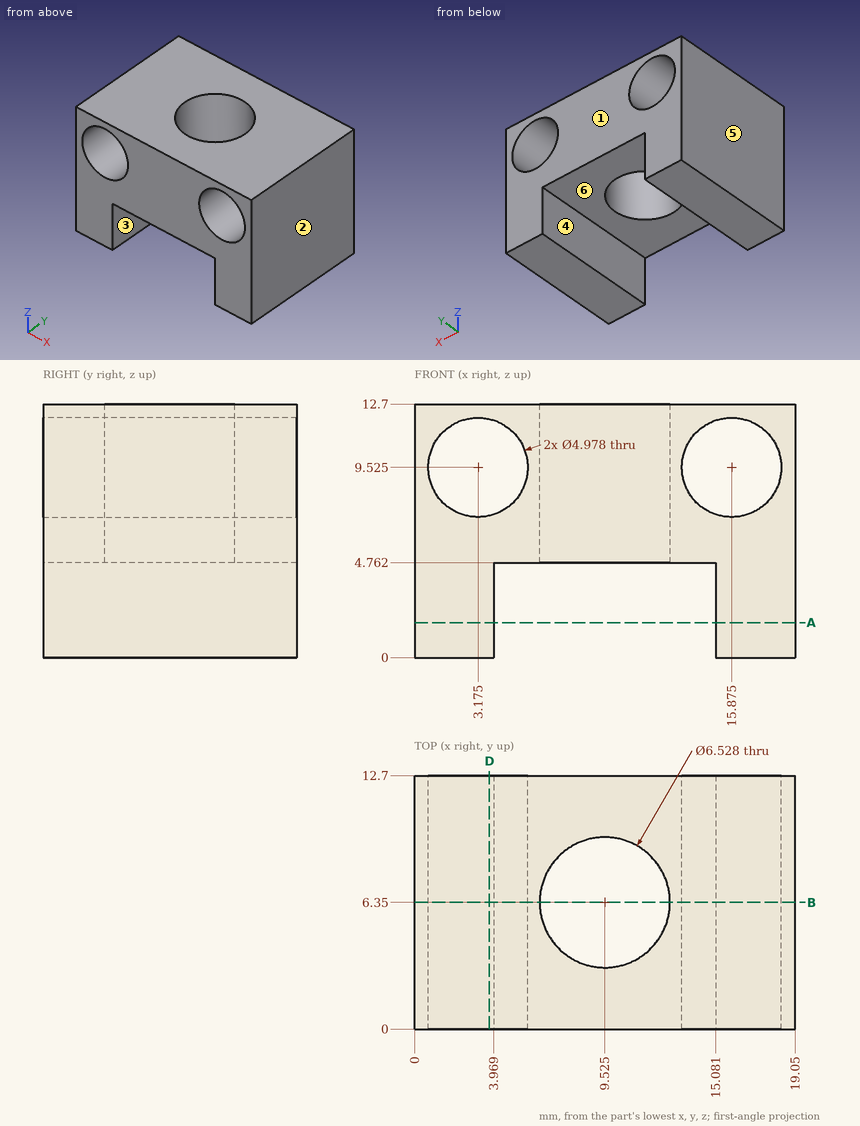
Geometry check sheet. Reference: drawing and pictorial views, mm from the part's lowest x, y, z. A direction names the side the tool comes from. Give positions to 0.01 mm unless a question says otherwise; leave off trailing zeros. Loops run counter-clockwise (first coordinate to the right, second up) from the corner with the lowest first, then second, coordinate; pieces in that order, holes last. Notation, with made-up numbers: M 6.25,-6 L 10.25,-6 A21 ccw 10.25,29 Z; hole C 44,12.5 d8. An arc over 180 degrees is marked long. Use a Markdown table: item, result. Add a question column.
Q1. Scan lines: line 1 along X through (y, z) = (1.5, 2.5); line 2 along Z through (x, y) = (11.5, 2.25); line 3 along Y through (x, z) = (7.5, 10.5). Record each from-to range of solid material in increasing order. Write a range as [from, to].
Q2. Mould release check, pull along X, two halves, no side actions. Record for the marked faces 1, 2, 3 and 4: pulls with the +X half, pulls with the -X half, needs draft (parallel to the pull), parting line crosses it, or undercut.
Q3. Sectioned sample at B-B, the plane y = 6.35. Give the number of separate pieces and of enclosed holes in the cut face.
Q4. Sectioned sample at D-D, the plane x = 3.75. Record the cut outline in (y, z).
Q5. Tool access check on the marked faces 5 and 6. Record the directions out of +Z, -Z, +X, -X, +Y, -Y that give a thin tool (end or side, any length) a straight path to the whole face; none if there is none.
Q6. Sectioned sample at A-A, the plane z = 1.75. Record the cut outline in (x, y), then the cut area to 3 significant figures.
Verdict:
| question | item | result |
|---|---|---|
| 1 | line 1 | [0, 3.97], [15.08, 19.05] |
| 1 | line 2 | [4.76, 12.7] |
| 1 | line 3 | [0, 3.79], [8.91, 12.7] |
| 2 | face 1 | needs draft |
| 2 | face 2 | pulls with the +X half |
| 2 | face 3 | undercut |
| 2 | face 4 | undercut |
| 3 | separate pieces | 2 |
| 3 | enclosed holes | 2 |
| 4 | outline | M 0,0 L 12.7,0 L 12.7,7.1 L 0,7.1 Z; M 0,11.95 L 12.7,11.95 L 12.7,12.7 L 0,12.7 Z |
| 5 | face 5 | +Z, -Z, -X, +Y, -Y |
| 5 | face 6 | -Z, +Y, -Y |
| 6 | outline | M 0,0 L 3.97,0 L 3.97,12.7 L 0,12.7 Z; M 15.08,0 L 19.05,0 L 19.05,12.7 L 15.08,12.7 Z |
| 6 | area | 101 mm^2 |
